Verification items for the finished model (mm, model axes). A direction names the side the tool comes from. Give positions to 0.01 mm unless a question says otherwise; leave off trailing zeros. Loops run counter-clockwise (first coordinate to the right, second up) from the corner with the lowest first, then second, coordinate; pieces in that order, holes last. Notation, with made-up numbers: (55, 79) - (110, 79) arc R18 cw to (110, 86) - close; hole circle Ø2 at (29, -27). An arc over 180 degrees is marked (long way). One line per item, written item: value. Start each with the question number.
1. Sectioned sample at A-A (z = -49). Record the cut outline in (x, y), plus the area to 3 significant figures.
2. Access from +Z, -Z, +X, -X, +Y, -Y to the whole of each face (thin tool, end or side, straight path). Record for faces 1 (the flat face through (-21, 0, 21)), 2 (the flat face through (-22.395, -0.493, -13.172)).
3. Mould release check, pull along X, two halves, no side actions. Record for faces 3 (the cylindrical face through (86.185, -0.507, -1.201)), 4 (the flat face through (6.404, -0.493, -48.908)), 5 (the flat face through (-21, -1, 21)), 6 (the cylindrical face through (-100.063, -0.493, -22.22)): pulls with the +X half, pulls with the -X half, needs draft (parallel to the pull), parting line crosses it, or undercut.
4. Gauge pin test, flat end, axial feed: pin 1 (2.5 mm diameter, centred on x = 32.5, z = 56.29, fed in from -Y). Record the tip position at first contact, or that the pin passes through.
5. Scan lines: L1, parallel to Z at x = 32.5, y = -0.45; L2, parallel to Z at x = -28, y = -0.45; L3, parallel to X at y = -0.45, z = -21. Record each from-to range of solid material in increasing order. Write a range as [from, to].
6. Sectioned sample at D-D (z = 34). Record the cut outline in (x, y).
7. Sectioned sample at C-C (y = -0.75). Count the separate pieces of the cut face and the enclosed holes in it, plus the area to 3 significant figures.
8. Sectioned sample at B-B (x = -78). Record the cut outline in (y, z).
from build123d import *

# Parameters (mm, degrees)
SKETCH_1_R               = 102.5
SM_BASE_FLANGE_1_DEPTH   = 1
HOLE_WIZARD_8_0_8_1_D    = 8
PATTERN_CIRCULAR_1_COUNT = 6
HOLE_WIZARD_3_3_3_3_1_D  = 3.3
HOLE_WIZARD_3_3_3_3_2_D  = 3.3
HOLE_WIZARD_3_3_3_3_3_D  = 3.3


# Sheet-metal steps are written as plain solids
with BuildPart() as part:
    # Sketch 1 → 基体-法兰1 (new body)
    with BuildSketch(Plane(origin=(0, 0, 0), x_dir=(1, 0, 0), z_dir=(0, 1, 0))):
        with Locations(Location((0, 0, 0), (0, 0, 270))):
            Circle(SKETCH_1_R)
        Polygon((-12.990381057, 37.5), (0, 60), (12.990381057, 37.5), (0, 45), align=None, mode=Mode.SUBTRACT)
        Polygon((30, 0), (15, 25.980762114), (-15, 25.980762114), (-30, 0), (-15, -25.980762114), (15, -25.980762114), align=None, mode=Mode.SUBTRACT)
    extrude(amount=-SM_BASE_FLANGE_1_DEPTH)

    # Ø8.0 (8) 直径孔1 (through all)
    with Locations(Plane(origin=(0, 0, 0), x_dir=(1, 0, 0), z_dir=(0, 1, 0))):
        with Locations((-45, 77.942286341)):
            hole_wizard_8_0_8_1 = Hole(HOLE_WIZARD_8_0_8_1_D / 2)

    # 阵列(圆周)1: Ø8.0 (8) 直径孔1 ×6 about axis
    pattern_circular_1_axis = Axis((0, 0, 0), (0, 1, 0))
    for i in range(1, PATTERN_CIRCULAR_1_COUNT):
        add(hole_wizard_8_0_8_1.rotate(pattern_circular_1_axis, i * 360 / PATTERN_CIRCULAR_1_COUNT), mode=Mode.SUBTRACT)

    # Ø3.3 (3.3) 直径孔1 (through all)
    with Locations(Plane(origin=(0, 0, 0), x_dir=(1, 0, 0), z_dir=(0, 1, 0))):
        with Locations((-48.5, 84.004464167), (-51.062177826, 74.442286341), (-41.5, 71.880108514), (-38.937822174, 81.442286341), (48.5, 84.004464167), (38.937822174, 81.442286341), (51.062177826, 74.442286341), (41.5, 71.880108514), (90, 7), (90, -7), (97, 0), (83, 0), (-83, 0), (-97, 0), (-90, 7), (-90, -7), (-48.5, -84.004464167), (-38.937822174, -81.442286341), (-41.5, -71.880108514), (-51.062177826, -74.442286341), (51.062177826, -74.442286341), (41.5, -71.880108514), (38.937822174, -81.442286341), (48.5, -84.004464167)):
            Hole(HOLE_WIZARD_3_3_3_3_1_D / 2)

    # Ø3.3 (3.3) 直径孔2 (through all)
    with Locations(Plane(origin=(0, 0, 0), x_dir=(1, 0, 0), z_dir=(0, 1, 0))):
        with Locations((32.5, -56.291651246), (65, 0), (32.5, 56.291651246), (-32.5, 56.291651246), (-65, 0), (-32.5, -56.291651246)):
            Hole(HOLE_WIZARD_3_3_3_3_2_D / 2)

    # Ø3.3 (3.3) 直径孔3 (through all)
    with Locations(Plane(origin=(0, 0, 0), x_dir=(1, 0, 0), z_dir=(0, 1, 0))):
        with Locations((0, 0), (27, -22), (-27, 22), (-27, -22), (27, 22)):
            Hole(HOLE_WIZARD_3_3_3_3_3_D / 2)


solid = part.part
Results are:
1. outline: (-90.03, -1) - (-6.35, -1) - (-6.35, 0) - (-90.03, 0) - close; (6.35, -1) - (90.03, -1) - (90.03, 0) - (6.35, 0) - close
1. area: 167 mm^2
2. face 1: +Z, -Z, +X, -X, +Y
2. face 2: +Y, -Y
3. face 3: undercut
3. face 4: undercut
3. face 5: needs draft
3. face 6: parting line crosses it
4. pin 1: passes through
5. L1: z = [-97.21, -57.94], [-54.64, 54.64], [57.94, 97.21]
5. L2: z = [-98.6, -23.31], [-20.69, -3.46], [3.46, 20.69], [23.31, 98.6]
5. L3: x = [-100.33, -28.31], [-25.69, -17.88], [17.88, 25.69], [28.31, 100.33]
6. outline: (-96.7, -1) - (96.7, -1) - (96.7, 0) - (-96.7, 0) - close
7. separate pieces: 1
7. enclosed holes: 42
7. area: 29,900 mm^2
8. outline: (-1, -66.5) - (0, -66.5) - (0, 66.5) - (-1, 66.5) - close
